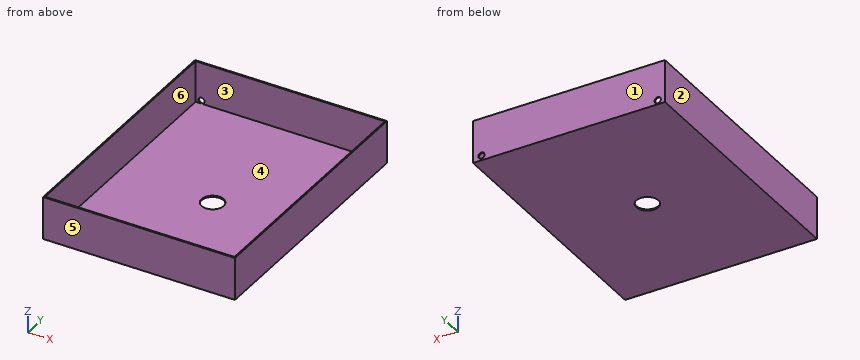
```python
from build123d import *

# Parameters (mm, degrees)
F0_W     = 914.4
F0_H     = 203.2
F1_DEPTH = 1219.2
F2_T     = -6.35
F3_R     = 14.923
F4_DEPTH = 6.35
F5_R     = 52.492005
F6_DEPTH = 6.351


with BuildPart() as f1:
    # F0 (on Front) → F1 (new body)
    with BuildSketch(Plane.XZ):
        with Locations((457.2, 101.6)):
            Rectangle(F0_W, F0_H)
    extrude(amount=F1_DEPTH)

    # F2
    f2_openings = [f1.faces().sort_by_distance(p)[0] for p in [
        (457.2, -609.6, 203.2),
    ]]
    offset(amount=F2_T, openings=f2_openings)

    # F3 (on face) → F4 (cut)
    with BuildSketch(Plane(origin=(0, 0, 0), x_dir=(-1, 0, 0), z_dir=(0, 1, 0))):
        with Locations((-874.310315, 23.554392)):
            Circle(F3_R)
        with Locations((-34.473307, 20.203399)):
            Circle(F3_R)
    extrude(amount=-F4_DEPTH, mode=Mode.SUBTRACT)

    # F5 (on face) → F6 (cut, through all)
    with BuildSketch(Plane.XY.offset(6.35)):
        with Locations((459.850729, -633.53318)):
            Circle(F5_R)
    extrude(amount=-F6_DEPTH, mode=Mode.SUBTRACT)


solid = f1.part
```
Build history of the part. All positions in model axes, mm. Face numbers are marked on the shaded views. A direction names the side the tool comes from. Coordinates: 2 decimals unless noted, no trailing zeros. Order: outer loops, then holes, each group sorted by start corner. A loop starts at its lowest first (then second) coordinate and runs counter-clockwise, first axis right, second up.
Item 1: Saw through at A-A on z = 156. List the corners of the cut face in (x, y), then the cut area to 3 significant figures.
Filled in:
outline: (0, -1219.2) - (914.4, -1219.2) - (914.4, 0) - (0, 0) - close; hole (6.35, -1212.85) - (908.05, -1212.85) - (908.05, -6.35) - (6.35, -6.35) - close
area: 26,900 mm2
Item 2: Drop flat-ended pins along their axis: pin 1 Ø10 at (x, y) = (779, -437) entering from +Z; pin 2 Ø8 at (y, z) = (-703, 154) entering from -X; pin 3 Ø0.5 at (x, z) = (33, 6) entering from +Y. Give the stop position or say it passes through.
Filled in:
pin 1: stops at z = 6.35
pin 2: stops at x = 0
pin 3: stops at y = -6.35
Item 3: Mould opens along Y. For the marked faces 1, 2, 3 and 4 say: released by +Y, released by -Y, zero draft, split by the parting line, or undercut.
Filled in:
face 1: released by +Y
face 2: zero draft
face 3: undercut
face 4: undercut
Item 4: Saw through at C-C on x = 749. List the corners of the cut face in (y, z).
Filled in:
outline: (-1219.2, 0) - (0, 0) - (0, 203.2) - (-6.35, 203.2) - (-6.35, 6.35) - (-1212.85, 6.35) - (-1212.85, 203.2) - (-1219.2, 203.2) - close
Item 5: Saw through at B-B on y = -1062.5. List the corners of the cut face in (x, z).
Filled in:
outline: (0, 0) - (914.4, 0) - (914.4, 203.2) - (908.05, 203.2) - (908.05, 6.35) - (6.35, 6.35) - (6.35, 203.2) - (0, 203.2) - close
Item 6: Drill centre lines: L1, parallel to Y at x = 499.5, z = 26.5; L2, parallel to X at y = -801.5, z = 188.5. Where is each one in solid material? Low to high.
Filled in:
L1: y = -1219.2 to -1212.85, -6.35 to 0
L2: x = 0 to 6.35, 908.05 to 914.4
Item 7: Tool access for the marked faces 5 and 6: list every direction of +Z, -Z, +X, -X, +Y, -Y with a clear straight run to the whole face (end or side of a thin tool).
Filled in:
face 5: +Z, -Z, +X, -X, -Y
face 6: +Z
